For this review, take the finished solid that the model builds, in its own axes (mm). A direction names the side the tool comes from. Round coordinates to 2 decimals unless told otherwise and drop trailing zeros. Loops run counter-clockwise (first coordinate to the right, second up) from the corner with the lowest first, then second, coordinate; pieces in that order, holes last. Notation, with made-up numbers: (-25, 55.5) -> (7, 55.5) arc R26 cw to (7, 85.5) -> close; hole circle Ø7 at (-39, 15). An arc over 180 degrees is marked (long way). Write each question's results on one line, items separated by ' | '.
```python
from build123d import *

# Parameters (mm, degrees)
F1_DEPTH = 17
F2_R     = 4.7
F3_DEPTH = 6
F4_R     = 19.4
F5_DEPTH = 3
F6_W     = 1.5
F6_H     = 1.7
F6_W_2   = 1.7
F6_H_2   = 1.5
F7_DEPTH = 55
F8_R     = 1


with BuildPart() as f1:
    # F0 (on Top) → F1 (new body)
    with BuildSketch(Plane.XY):
        Polygon((3.875, -2.2372322931), (3.875, 2.2372322931), (0, 4.4744645862), (-3.875, 2.2372322931), (-3.875, -2.2372322931), (0, -4.4744645862), align=None)
    extrude(amount=-F1_DEPTH)

    # F2 (on face) → F3 (join)
    with BuildSketch(Plane.XY):
        Circle(F2_R)
    extrude(amount=F3_DEPTH)

    # F4 (on face) → F5 (join)
    with BuildSketch(Plane.XY.offset(6)):
        Circle(F4_R)
    extrude(amount=F5_DEPTH)

    # F6 (on face) → F7 (join)
    with BuildSketch(Plane.XY.offset(9)):
        with Locations((-1.6, 0)):
            Rectangle(F6_W, F6_H)
        with Locations((0, 1.6)):
            Rectangle(F6_W_2, F6_H_2)
        Rectangle(F6_W_2, F6_H)
        with Locations((1.6, 0)):
            Rectangle(F6_W, F6_H)
        with Locations((0, -1.6)):
            Rectangle(F6_W_2, F6_H_2)
    extrude(amount=F7_DEPTH)

    # F8
    f8_edges = [f1.edges().sort_by_distance(p)[0] for p in [
        (-19.4, 0, 6),
        (-19.4, 0, 9),
    ]]
    fillet(f8_edges, radius=F8_R)


solid = f1.part
```
1. Tool access review of faces 1 (the face through (-3.875, 0, -8)), 2 (the face through (-1.02, -4.59, 2.96)), 3 (the face through (-0.85, 2, 36)), 4 (the face through (0.85, -2, 36)), 5 (the face through (-2, -0.85, 36)): name each direction out of +Z, -Z, +X, -X, +Y, -Y from which nothing blocks a thin tool from reaching the whole face with its end or side.
Values found:
face 1: -Z, -X, +Y, -Y | face 2: -Z | face 3: +Z, -X, +Y | face 4: +Z, +X, -Y | face 5: +Z, -X, -Y
2. Consider section A-A (z = 12.5). State the section outline as (x, y) points.
Values found:
outline: (-2.35, -0.85) -> (-0.85, -0.85) -> (-0.85, -2.35) -> (0.85, -2.35) -> (0.85, -0.85) -> (2.35, -0.85) -> (2.35, 0.85) -> (0.85, 0.85) -> (0.85, 2.35) -> (-0.85, 2.35) -> (-0.85, 0.85) -> (-2.35, 0.85) -> close
3. Consider section B-B (y = 0). State the section outline as (x, z) points (3 decimals).
Values found:
outline: (-19.4, 7) arc R1 ccw to (-18.4, 6) -> (-4.7, 6) -> (-4.7, 0) -> (-3.875, 0) -> (-3.875, -17) -> (3.875, -17) -> (3.875, 0) -> (4.7, 0) -> (4.7, 6) -> (18.4, 6) arc R1 ccw to (19.4, 7) -> (19.4, 8) arc R1 ccw to (18.4, 9) -> (2.35, 9) -> (2.35, 64) -> (-2.35, 64) -> (-2.35, 9) -> (-18.4, 9) arc R1 ccw to (-19.4, 8) -> close
4. To check wall thickness, follow probe 1 along Z at (x, y) = (-12, 2.5); probe 2 along Y at (x, z) = (0.5, 57.5); probe 3 along Z at (x, y) = (-3, 2). State the ranges of each line that lie inside material, in increasing order.
Values found:
probe 1: z = 6 to 9 | probe 2: y = -2.35 to 2.35 | probe 3: z = -17 to 9
5. For pin 1 (1.4 mm diameter, centred on y = 0, z = 38, fed in from +X); pin 2 (3.5 mm diameter, centred on y = 0, z = -6, fed in from -X) (3 decimals); pin 3 (0.5 mm diameter, centred on y = 0, z = 39.5, fed in from -X), all flat-tipped, find the tip position at first contact; note any pin that passes through.
Values found:
pin 1: stops at x = 2.35 | pin 2: stops at x = -3.875 | pin 3: stops at x = -2.35
